Design review of the part built by this model. Coordinates are the model's own, in mm. Coordinates: 2 decimals unless noted, no trailing zeros. Loops run counter-clockwise (first coordinate to the right, second up) from the corner with the lowest first, then second, coordinate; pieces in that order, holes last.
from build123d import *

# Parameters (mm, degrees)
SKETCH1_R           = 2.45745
BOSS_EXTRUDE1_DEPTH = 12.7
FILLET1_R           = 3.175


with BuildPart() as part:
    # Sketch1 → Boss-Extrude1 (new body)
    with BuildSketch(Plane(origin=(0, 0, 0), x_dir=(1, 0, 0), z_dir=(0, 1, 0))):
        Polygon((-0.199185023, -544.98942083), (472.075100704, -272.319932268), (472.075100704, -189.70625), (472.075100704, -89.69375), (472.075100704, 0), (0, 0), (-236.036311861, -408.829744745), (-159.04651881, -453.279511515), (-71.058183894, -504.079244967), align=None)
        with Locations((-169.646411276, -357.338592529)):
            Circle(SKETCH1_R, mode=Mode.SUBTRACT)
        with Locations((-18.164146109, -94.961777227)):
            Circle(SKETCH1_R, mode=Mode.SUBTRACT)
        with Locations((91.321480704, -31.749605568)):
            Circle(SKETCH1_R, mode=Mode.SUBTRACT)
        with Locations((394.287600704, -31.749605568)):
            Circle(SKETCH1_R, mode=Mode.SUBTRACT)
        with Locations((384.876900704, -271.337645568)):
            Circle(SKETCH1_R, mode=Mode.SUBTRACT)
        with Locations((213.713214706, -370.159699049)):
            Circle(SKETCH1_R, mode=Mode.SUBTRACT)
        with Locations((42.549528708, -468.981752529)):
            Circle(SKETCH1_R, mode=Mode.SUBTRACT)
    extrude(amount=BOSS_EXTRUDE1_DEPTH)

    # Fillet1
    fillet1_edges = [part.edges().sort_by_distance(p)[0] for p in [
        (472.075100704, 6.35, 272.319932268),
        (-0.199185023, 6.35, 544.98942083),
        (-236.036311861, 6.35, 408.829744745),
        (0, 6.35, 0),
        (472.075100704, 6.35, 0),
    ]]
    fillet(fillet1_edges, radius=FILLET1_R)


solid = part.part
Q1. Clearance check with flat-ended pins moving along their axes: pin 1 Ø2 at (x, y) = (-96, 6.5) entering from +Z; pin 2 Ø3 at (y, z) = (2.5, 309) entering from +X; pin 3 Ø2 at (y, z) = (2, 120) entering from -X. State where each tip first meets the part, or that it passes through.
Q2. Take a section at B-B, the plane x = 362.5. Write out the cut boundary in (y, z).
Q3. Take a section at C-C, the plane z = 303. Write out the cut boundary in (x, y).
Q4. Take a section at A-A, the plane y = 4.5. Give the number of separate pieces and of enclosed holes in the cut face, then the cut area to 3 significant figures.
Q5. For line 1 (X direction, y = 9.75, z = 192); line 2 (Z direction, x = 37, y = 10.75); line 3 (X direction, y = 8.75, z = 186.5), list the stretches that pass through material, from the lowest coordinate up.
Entries:
1. pin 1: stops at z = 490.26
1. pin 2: stops at x = 411.14
1. pin 3: stops at x = -69.86
2. outline: (0, 0) - (12.7, 0) - (12.7, 335.58) - (0, 335.58) - close
3. outline: (-174.94, 0) - (418.94, 0) - (418.94, 12.7) - (-174.94, 12.7) - close
4. separate pieces: 1
4. enclosed holes: 7
4. area: 257,000 mm2
5. line 1: x = -110.85 to 472.08
5. line 2: z = 0 to 523.51
5. line 3: x = -107.68 to 472.08
